Read the model definition and answer for the solid it produces. Units are mm, in the model's axes. A direction names the side the tool comes from. Round coordinates to 2 decimals unless told otherwise and drop trailing zeros. Order: outer loops, then holes, each group sorted by start corner. A loop starts at its lowest first (then second) coordinate and runs counter-clockwise, first axis right, second up. Notation, with made-up numbers: (71, 51) -> (97, 51) arc R29 cw to (97, 75) -> close; hole circle Ø4 at (-19, 52.5). An arc over 180 degrees is marked (long way). Use a Markdown table: item, result. Add a question column.
1. The mould has two halves that part along X. Classify faces 4 (the face through (10, -4, 10)), 5 (the face through (-0.43, -3, 10)), 6 (the face through (0, -15, -7)), 7 (the face through (0.496, -4, 10)): +X half, -X half, draft (parallel to the pull), parting line (faces both ways), or undercut.
2. Given pin 1 (2 mm diameter, centred on x = -2, y = -7, fed in from -Z); pin 2 (6.5 mm diameter, centred on y = -5, z = 11, fed in from +X); pin 3 (5.5 mm diameter, centred on x = 5.5, z = 8, fed in from -Y); pin 4 (2 mm diameter, centred on x = -4, z = 6.5, fed in from +Y), each flat-ended and moving along its own axis, determine where each tip first touches the part or whether it passes through.
3. Section D-D, the plane y = -0.75 is taken. Give the vertices of the cut face in (x, z).
4. For faces 1 (the face through (6, -6.903, 9)), 2 (the face through (-6.207, -10.895, 3.838)), 3 (the face through (-6, -6.903, 9)), determine the directions among +Z, -Z, +X, -X, +Y, -Y from which every point of the face is accessible in a straight line to the end or side of a thin tool.
5. Consider L1, parallel to X at y = -9, z = 0; L2, parallel to Z at x = 2.5, y = -1.25; L3, parallel to Y at x = -8, z = 5.75. Determine where each line is inside the solid, lowest interval first. Write a range as [from, to].
```python
from build123d import *

# Parameters (mm, degrees)
SKETCH_R             = 10
SKETCH_R_2           = 6.5
PAD_DEPTH            = 15
POCKET_DEPTH         = 15
POCKET_DEPTH_BACK    = -15
PAD001_DEPTH         = 10
PAD001_DEPTH_BACK    = 10
SKETCH003_W          = 0.925108
SKETCH003_H          = 21.969815
POCKET001_DEPTH      = 15
POCKET001_DEPTH_BACK = -15
SKETCH004_R          = 6.5
POCKET002_DEPTH      = 15
POCKET002_DEPTH_BACK = -15


with BuildPart() as part:
    # Sketch (on XZ_Plane of Origin) → Pad (new body)
    with BuildSketch(Plane.XZ):
        with Locations((0.223041, 0)):
            Circle(SKETCH_R)
        Circle(SKETCH_R_2, mode=Mode.SUBTRACT)
    extrude(amount=PAD_DEPTH)

    # Sketch001 (on YZ_Plane of Origin) → Pocket (cut, two sides)
    with BuildSketch(Plane.YZ) as pocket_sk:
        Polygon((-5.152612, 12.624485), (-17.571489, -6.377891), (-30.254476, 15.01538), (-10.204725, 21.22482), align=None)
    extrude(amount=-POCKET_DEPTH, mode=Mode.SUBTRACT)
    extrude(pocket_sk.sketch, amount=-POCKET_DEPTH_BACK, mode=Mode.SUBTRACT)

    # Sketch002 (on YZ_Plane of Origin) → Pad001 (join, two sides)
    with BuildSketch(Plane.YZ) as pad001_sk:
        with BuildLine():
            ThreePointArc((-0.00519, 11.247658), (-3.454061, 14.696529), (-6.902933, 11.247658))
            Line((-6.902933, 11.247658), (-6.902933, 4.5552))
            Line((-0.00519, 4.5552), (-6.902933, 4.5552))
            Line((-0.00519, 11.247658), (-0.00519, 4.5552))
        make_face()
    extrude(amount=PAD001_DEPTH)
    extrude(pad001_sk.sketch, amount=-PAD001_DEPTH_BACK)

    # Sketch003 (on XZ_Plane of Origin) → Pocket001 (cut, two sides)
    with BuildSketch(Plane.XZ) as pocket001_sk:
        with Locations((0.033004, 12.288593)):
            Rectangle(SKETCH003_W, SKETCH003_H)
    extrude(amount=-POCKET001_DEPTH, mode=Mode.SUBTRACT)
    extrude(pocket001_sk.sketch, amount=-POCKET001_DEPTH_BACK, mode=Mode.SUBTRACT)

    # Sketch004 (on XZ_Plane of Origin) → Pocket002 (cut, two sides)
    with BuildSketch(Plane.XZ) as pocket002_sk:
        Circle(SKETCH004_R)
    extrude(amount=-POCKET002_DEPTH, mode=Mode.SUBTRACT)
    extrude(pocket002_sk.sketch, amount=-POCKET002_DEPTH_BACK, mode=Mode.SUBTRACT)


solid = part.part
```
Verdict:
| question | item | result |
|---|---|---|
| 1 | face 4 | +X half |
| 1 | face 5 | undercut |
| 1 | face 6 | draft |
| 1 | face 7 | undercut |
| 2 | pin 1 | stops at z = -9.92 |
| 2 | pin 2 | stops at x = 10 |
| 2 | pin 3 | stops at y = -9.97 |
| 2 | pin 4 | stops at y = 0 |
| 3 | outline | (-10, 4.56) -> (-8.68, 4.56) arc R10 ccw (long way) to (9.13, 4.56) -> (10, 4.56) -> (10, 13.39) -> (0.5, 13.39) -> (0.5, 6.48) arc R6.5 cw (long way) to (-0.43, 6.49) -> (-0.43, 13.39) -> (-10, 13.39) -> close |
| 4 | face 1 | +Z, +X, -Y |
| 4 | face 2 | +Z, +X, -X, -Y |
| 4 | face 3 | +Z, -X, -Y |
| 5 | L1 | x = [-9.78, -6.5], [6.5, 10.22] |
| 5 | L2 | z = [-9.74, -6], [6, 13.9] |
| 5 | L3 | y = [-6.9, -0.01] |
